Read the model definition and answer for the solid it produces. Units are mm, in the model's axes. Face numbers are marked on the shaded views. A direction names the side the tool comes from. Coordinates: 2 decimals unless noted, no trailing zeros. Loops run counter-clockwise (first coordinate to the right, second up) from the corner with the lowest first, then second, coordinate; pieces in that order, holes last. Notation, with made-up numbers: (-18.5, -33) -> (32.5, -33) arc R29 cw to (32.5, -12) -> close; hole circle Ø1 at (-14.5, 24). An arc over 180 degrees is marked (long way). Answer as a JSON object with one key per item and string values. Group by question number.
Q1. Straight lines are drawn through the part: line 1 along Z through (x, y) = (-7.5, -11); line 2 along Y through (x, z) = (-17.5, -20); line 3 along Y through (x, z) = (-5.5, 11). For each, find the intervals that lie inside material, in ascending order. Write a range as [from, to].
Q2. Determine the mould class of the marked faces 4, 5, 6 and 7 for opening direction Z: released by +Z, released by -Z, zero draft, split by the parting line, or undercut.
Q3. Each of these flat-tipped pins is pushed along its axis until it touches: P1, Ø10, axis at x = 11, z = 17.5, coming from the +Y side; P2, Ø8, axis at y = 33, z = -1, coming from the +X side; P3, Ø1, axis at x = -23, z = -7.5, coming from the +Y side; P4, Ø4, axis at x = 17.5, y = -20, coming from the -Z side. Where does it stop, or does it pass through?
Q4. The part is cut by section D-D on y = -4. Write down the section's boundary in (x, z), and give its area (3 significant figures).
Q5. For the marked faces 1, 2 and 3, determine the directions among +Z, -Z, +X, -X, +Y, -Y from which every point of the face is accessible in a straight line to the end or side of a thin tool.
Q6. The part is cut by section B-B on x = 23. Write down the section's boundary in (y, z), and give its area (3 significant figures).
Q7. The part is cut by section A-A on y = -20. Write down the section's boundary in (x, z).
Q8. The part is cut by section C-C on z = 0. Write down the section's boundary in (x, y).
from build123d import *

# Parameters (mm, degrees)
SKETCH1_W           = 60
SKETCH1_H           = 46
BOSS_EXTRUDE1_DEPTH = 10
SKETCH2_W           = 60
SKETCH2_H           = 10
BOSS_EXTRUDE2_DEPTH = 40
SKETCH3_R           = 18
BOSS_EXTRUDE3_DEPTH = 40
SKETCH4_R           = 2.5
CUT_EXTRUDE1_DEPTH  = 75.269778511


with BuildPart() as part:
    # Sketch1 → Boss-Extrude1 (new body)
    with BuildSketch(Plane(origin=(0, 0, 0), x_dir=(1, 0, 0), z_dir=(0, 1, 0))):
        Rectangle(SKETCH1_W, SKETCH1_H)
    extrude(amount=BOSS_EXTRUDE1_DEPTH)

    # Sketch2 → Boss-Extrude2 (add)
    with BuildSketch(Plane.XZ):
        with Locations((0, 18)):
            Rectangle(SKETCH2_W, SKETCH2_H)
        with Locations((0, -18)):
            Rectangle(SKETCH2_W, SKETCH2_H)
    extrude(amount=BOSS_EXTRUDE2_DEPTH)

    # Sketch3 → Boss-Extrude3 (add)
    with BuildSketch(Plane(origin=(0, 10, 0), x_dir=(1, 0, 0), z_dir=(0, 1, 0))):
        with Locations(Location((0, 0, 0), (0, 0, 270))):
            Circle(SKETCH3_R)
    extrude(amount=BOSS_EXTRUDE3_DEPTH)

    # Sketch4 → Cut-Extrude1 (cut, through all)
    with BuildSketch(Plane(origin=(0, 0, -23), x_dir=(-1, 0, 0), z_dir=(0, 0, -1))):
        with Locations((-17.5, -20)):
            Circle(SKETCH4_R)
        with Locations((17.5, -20)):
            Circle(SKETCH4_R)
    extrude(amount=-CUT_EXTRUDE1_DEPTH, mode=Mode.SUBTRACT)


solid = part.part
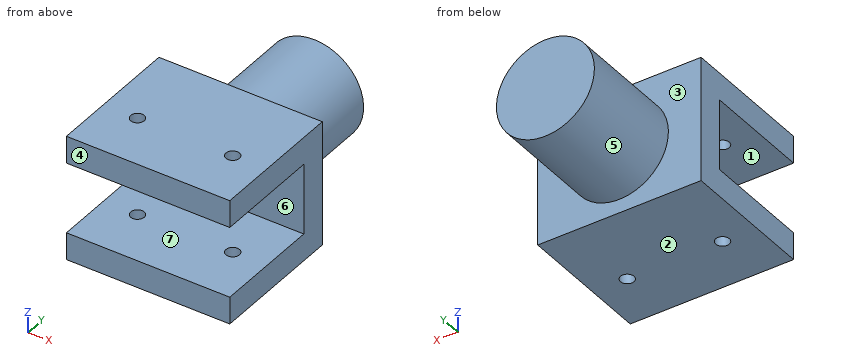
Final values:
{
 "1": {"line 1": "z = [-23, -13], [13, 23]", "line 2": "y = [-40, -22.5], [-17.5, 10]", "line 3": "y = [0, 50]"},
 "2": {"face 4": "zero draft", "face 5": "split by the parting line", "face 6": "undercut", "face 7": "undercut"},
 "3": {"P1": "stops at y = 50", "P2": "stops at x = 18", "P3": "stops at y = 10", "P4": "passes through"},
 "4": {"outline": "(-30, -23) -> (30, -23) -> (30, -13) -> (-30, -13) -> close; (-30, 13) -> (30, 13) -> (30, 23) -> (-30, 23) -> close", "area": "1,200 mm2"},
 "5": {"face 1": "+X, -X, -Y", "face 2": "-Z, +X, -X, +Y, -Y", "face 3": "+Y"},
 "6": {"outline": "(-40, -23) -> (10, -23) -> (10, 23) -> (-40, 23) -> (-40, 13) -> (0, 13) -> (0, -13) -> (-40, -13) -> close", "area": "1,260 mm2"},
 "7": {"outline": "(-30, -23) -> (-20, -23) -> (-20, -13) -> (-30, -13) -> close; (-30, 13) -> (-20, 13) -> (-20, 23) -> (-30, 23) -> close; (-15, -23) -> (15, -23) -> (15, -13) -> (-15, -13) -> close; (-15, 13) -> (15, 13) -> (15, 23) -> (-15, 23) -> close; (20, -23) -> (30, -23) -> (30, -13) -> (20, -13) -> close; (20, 13) -> (30, 13) -> (30, 23) -> (20, 23) -> close"},
 "8": {"outline": "(-30, 0) -> (30, 0) -> (30, 10) -> (18, 10) -> (18, 50) -> (-18, 50) -> (-18, 10) -> (-30, 10) -> close"}
}
